The drawing under review shows one solid part. Ordinate dimensions are in mm from its lowest x, y, z. Give positions to 0.01 mm unless a question says otherwise; leave off trailing zeros. Write each loop counter-clockwise with the first axis right and the second up, starting at its lowest first coordinate (ties: lowest second). Pieces come first, ordered by that corner, then holes.
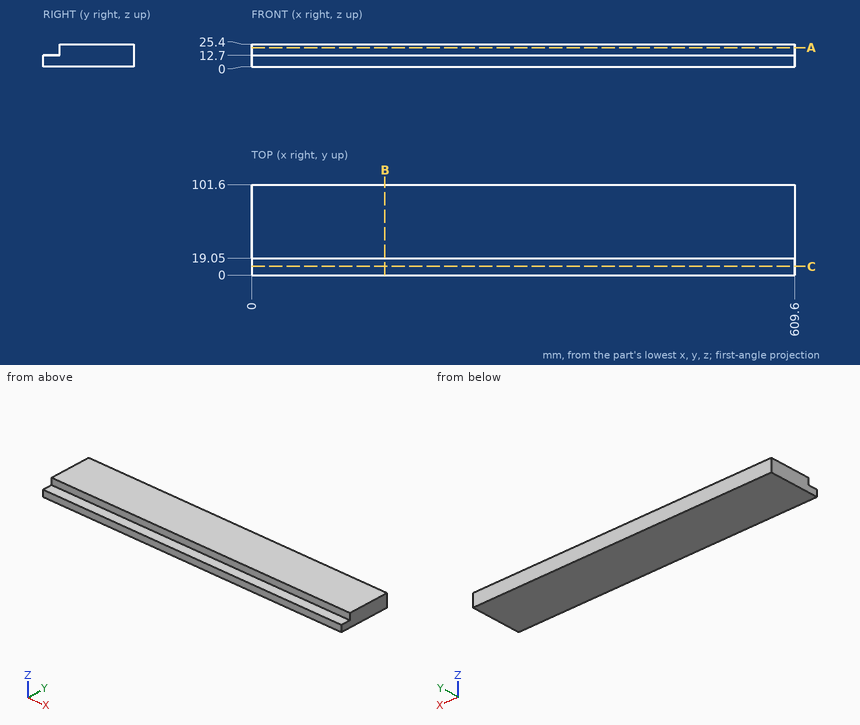
1) Insertion check: pin 1 (1 mm diameter, centred on y = 18.5, z = 16.5, fed in from -X); pin 2 (4 mm diameter, centred on x = 344.5, z = 20.5, fed in from -Y); pin 3 (21 mm diameter, centred on x = 408, y = 11.5, fed in from +Z). Each pin has a flat end and moves straight along its axis. Give the tip position at first contact, or say it passes through.
2) Consider section A-A, the plane z = 21.25. Give the boundary of the cut face in (x, y).
3) Consider section B-B, the plane x = 149.5. Give the boundary of the cut face in (y, z), then the cut area to 3 significant figures.
4) To check wall thickness, follow probe 1 along Z at (x, y) = (508, 7); probe 2 along Y at (x, z) = (497, 14.5). State the ranges of each line that lie inside material, in increasing order.
5) Consider section C-C, the plane y = 10. Give the boundary of the cut face in (x, z), then the cut area to 3 significant figures.
Answer block:
1. pin 1: passes through
1. pin 2: stops at y = 19.05
1. pin 3: stops at z = 25.4
2. outline: (0, 19.05) - (609.6, 19.05) - (609.6, 101.6) - (0, 101.6) - close
3. outline: (0, 0) - (101.6, 0) - (101.6, 25.4) - (19.05, 25.4) - (19.05, 12.7) - (0, 12.7) - close
3. area: 2,340 mm2
4. probe 1: z = 0 to 12.7
4. probe 2: y = 19.05 to 101.6
5. outline: (0, 0) - (609.6, 0) - (609.6, 12.7) - (0, 12.7) - close
5. area: 7,740 mm2
